from build123d import *

# Parameters (mm, degrees)
SALIENTE_EXTRUIR1_DEPTH = 10
CROQUIS2_R              = 1
CORTAR_EXTRUIR1_DEPTH   = 10


with BuildPart() as part:
    # Croquis1 → Saliente-Extruir1 (new body)
    with BuildSketch(Plane.XY):
        with BuildLine():
            Line((12.5, -2), (6, -2))
            ThreePointArc((6, -2), (0, 4), (-6, -2))
            Line((-6, -2), (-12.5, -2))
            Line((-12.5, -2), (-12.5, 2))
            Line((-12.5, 2), (-8.062257748, 2))
            ThreePointArc((-8.062257748, 2), (0, 7), (8.062257748, 2))
            Line((8.062257748, 2), (12.5, 2))
            Line((12.5, 2), (12.5, -2))
        make_face()
    extrude(amount=SALIENTE_EXTRUIR1_DEPTH)

    # Croquis2 → Cortar-Extruir1 (cut)
    with BuildSketch(Plane(origin=(0, 2, 0), x_dir=(1, 0, 0), z_dir=(0, 1, 0))):
        with Locations(Location((10.5, -5, 0), (0, 0, 180))):
            Circle(CROQUIS2_R)
    cortar_extruir1 = extrude(amount=-CORTAR_EXTRUIR1_DEPTH, mode=Mode.SUBTRACT)

    # Simetría1: Cortar-Extruir1 across plane
    add(cortar_extruir1.mirror(Plane(origin=(0, 0, 0), x_dir=(0, 0, 1), z_dir=(1, 0, 0))), mode=Mode.SUBTRACT)


solid = part.part
Could you check a few things on this model? Use its own coordinates, in mm. A direction names the side the tool comes from. Coordinates: 2 decimals unless noted, no trailing zeros. Write each loop counter-clockwise with the first axis right and the second up, starting at its lowest first coordinate (ties: lowest second). Pieces come first, ordered by that corner, then holes. Notation, with made-up numbers: (81.5, 64.5) - (112.5, 64.5) arc R23 ccw to (112.5, 77.5) - close; hole circle Ø4 at (73.5, -20). An arc over 180 degrees is marked (long way). Write item = value, one per line.
1) Will these pins go through, and if not, where does the flat tip stop? pin 1 Ø1 at (x, z) = (-1, 1.5) entering from +Y; pin 2 Ø2 at (x, z) = (9.5, 5) entering from +Y; pin 3 Ø1 at (x, z) = (1.5, 8) entering from +Y; pin 4 Ø1.6 at (x, z) = (-10.5, 5) entering from -Y.
Result set:
pin_1 = 6.99
pin_2 = 2
pin_3 = 6.94
pin_4 = through
2) Suppose I cut it at B-B on y = 3.25. Please give me the cut outline in (x, z).
Result set:
outline = (-7.31, 0) - (-2.9, 0) - (-2.9, 10) - (-7.31, 10) - close; (2.9, 0) - (7.31, 0) - (7.31, 10) - (2.9, 10) - close
3) We'd pull the mould along Z, two halves only. Please class faces 1 (the cylindrical face through (11.237, 0.028, 5.676)), 2 (the flat face through (9, 2, 5)), 3 (the flat face through (0, 5, 10)): +Z half, -Z half, draft (parallel to the pull), parting line (faces both ways), or undercut.
Result set:
face_1 = undercut
face_2 = draft
face_3 = +Z half
4) Please list where these lines run through material, in increasing order: line 1 (Z direction, x = 10.5, y = 0.6); line 2 (Y direction, x = -9, z = 5.75); line 3 (X direction, y = 1.75, z = 7.75). Write a range as [from, to].
Result set:
line_1 = [0, 4], [6, 10]
line_2 = [-2, 2]
line_3 = [-12.5, -4.68], [4.68, 12.5]
5) Suppose I cut it at C-C on x = 10.5. Please give me the cut outline in (y, z), plus the area to 3 significant figures.
Result set:
outline = (-2, 0) - (2, 0) - (2, 4) - (-2, 4) - close; (-2, 6) - (2, 6) - (2, 10) - (-2, 10) - close
area = 32.0 mm2
6) Suppose I cut it at A-A on z = 5. Please give me the cut outline in (x, y), plus the area to 3 significant figures.
Result set:
outline = (-12.5, -2) - (-11.5, -2) - (-11.5, 2) - (-12.5, 2) - close; (-9.5, -2) - (-6, -2) arc R6 cw to (6, -2) - (9.5, -2) - (9.5, 2) - (8.06, 2) arc R9 ccw to (-8.06, 2) - (-9.5, 2) - close; (11.5, -2) - (12.5, -2) - (12.5, 2) - (11.5, 2) - close
area = 85.1 mm2
7) Suppose I cut it at D-D on y = 1.25. Please give me the cut outline in (x, z), plus the area to 3 significant figures.
Result set:
outline = (-12.5, 0) - (-5.04, 0) - (-5.04, 10) - (-12.5, 10) - close; (5.04, 0) - (12.5, 0) - (12.5, 10) - (5.04, 10) - close; hole circle Ø2 at (-10.5, 5); hole circle Ø2 at (10.5, 5)
area = 143 mm2
8) For faces 4 (the flat face through (9, -2, 5)), 5 (the flat face through (-9, 2, 5)), which set-ups out of +Z, -Z, +X, -X, +Y, -Y let a thin tool reach every point of the face, with its end or its side?
Result set:
face_4 = +Z, -Z, +X, -X, -Y
face_5 = +Z, -Z, -X, +Y
